Input: part model. Units: mm. Frame: model coordinates. Face numbers are marked on the shaded views. A direction names the side the tool comes from. Round coordinates to 2 decimals unless told otherwise and drop trailing zeros. Loops run counter-clockwise (first coordinate to the right, second up) from the corner with the lowest first, then second, coordinate; pieces in that order, holes last. Notation, with made-up numbers: (20, 72.5) - (64, 72.5) arc R16 ccw to (64, 81.5) - close; hole circle Ø7 at (80.25, -10.75). An arc over 180 degrees is marked (long way). Use CSV: the item, a comma, the result in double quotes. Start each with the question number.
1. Material intervals for probe 1 along X at (y, z) = (-58, 121.5); probe 2 along Y at (x, z) = (34.5, 263); probe 3 along Z at (x, y) = (143, -280.5), sorted ascending. Write a range as from..to.
2. Cut plane B-B (y = -93.5). Return loops of the section in (x, z) (3 decimals).
3. Pin query (flat end, axial travel): P1, Ø5, axis at x = 423.5, y = -401, coming from the +Z side; P2, Ø1, axis at y = -327.5, z = 31, coming from the -X side; P3, Ø5.5, axis at y = -265, z = 11, coming from the +X side. Return the tip coordinate at first contact, or that it passes through.
4. Pull-direction query (X, two-part tool) for the marked faces 1, 2 and 3; classes: +X half, -X half, draft (parallel to the pull), parting line (faces both ways), or undercut.
5. Cut plane C-C (x = 41). Return loops of the section in (y, z) (3 decimals).
6. Access query for the marked faces 4, 5 and 6. Directions: +Z, -Z, +X, -X, +Y, -Y. A direction counts if a zero-diameter tool reaches every point of the face in a straight line with its end or side. Return the directions, or none.
7. Cut plane A-A (z = 38.5). Return loops of the section in (x, y).
```python
from build123d import *

# Parameters (mm, degrees)
F0_W     = 520.7
F0_H     = 347.345
F1_DEPTH = 914.4
F2_T     = -11.90625
F4_DEPTH = 6.35
F5_W     = 496.8875
F5_H     = 3.175
F6_DEPTH = 366.396
F7_W     = 503.2375
F7_H     = 8.73125
F8_DEPTH = 914.4


with BuildPart() as f1:
    # F0 (on Front) → F1 (new body)
    with BuildSketch(Plane.XZ):
        with Locations((260.35, 173.6725)):
            Rectangle(F0_W, F0_H)
    extrude(amount=F1_DEPTH)

    # F2
    f2_openings = [f1.faces().sort_by_distance(p)[0] for p in [
        (260.35, -457.2, 347.345),
        (260.35, -457.2, 0),
    ]]
    offset(amount=F2_T, openings=f2_openings)

    # F3 (on face) → F4 (join)
    with BuildSketch(Plane.XZ.offset(914.4)):
        with BuildLine():
            ThreePointArc((-19.05, -6.35), (-15.330256, -15.330256), (-6.35, -19.05))
            Line((-6.35, -19.05), (527.05, -19.05))
            ThreePointArc((527.05, -19.05), (536.030256, -15.330256), (539.75, -6.35))
            Line((539.75, -6.35), (539.75, 353.695))
            ThreePointArc((539.75, 353.695), (536.030256, 362.675256), (527.05, 366.395))
            Line((527.05, 366.395), (-6.35, 366.395))
            ThreePointArc((-6.35, 366.395), (-15.330256, 362.675256), (-19.05, 353.695))
            Line((-19.05, 353.695), (-19.05, -6.35))
        make_face()
    extrude(amount=F4_DEPTH)

    # F5 (on face) → F6 (cut, through all)
    with BuildSketch(Plane.XY.offset(347.345)):
        with Locations((260.35, -10.31875)):
            Rectangle(F5_W, F5_H)
    extrude(amount=-F6_DEPTH, mode=Mode.SUBTRACT)

    # F7 (on face) → F8 (join, through all)
    with BuildSketch(Plane(origin=(0, 0, 0), x_dir=(-1, 0, 0), z_dir=(0, 1, 0))):
        with Locations((-260.35, 23.415625)):
            Rectangle(F7_W, F7_H)
    extrude(amount=-F8_DEPTH)


solid = f1.part
```
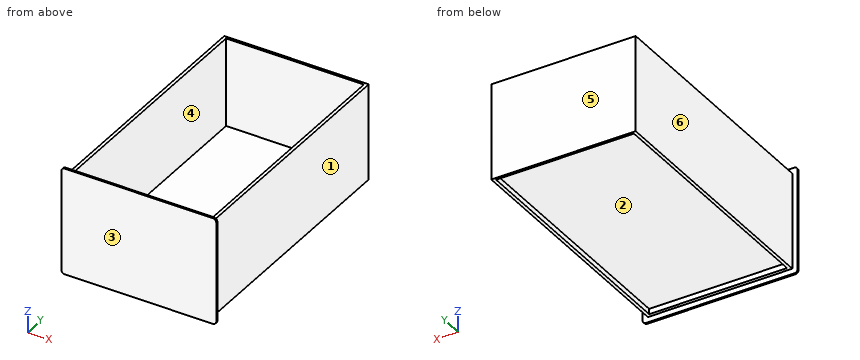
Established:
1,probe 1,"x = 0..11.91, 508.79..520.7"
1,probe 2,"y = -920.75..-902.49, -8.73..0"
1,probe 3,"z = 19.05..27.78"
2,outline,"(0, 0) - (11.906, 0) - (11.906, 19.05) - (508.794, 19.05) - (508.794, 0) - (520.7, 0) - (520.7, 347.345) - (508.794, 347.345) - (508.794, 27.781) - (11.906, 27.781) - (11.906, 347.345) - (0, 347.345) - close"
3,P1,"stops at z = 27.78"
3,P2,"stops at x = 0"
3,P3,"stops at x = 520.7"
4,face 1,"+X half"
4,face 2,"undercut"
4,face 3,"draft"
5,outline,"(-920.75, -19.05) - (-914.4, -19.05) - (-914.4, 0) - (-902.494, 0) - (-902.494, 19.05) - (-8.731, 19.05) - (-8.731, 0) - (0, 0) - (0, 347.345) - (-8.731, 347.345) - (-8.731, 27.781) - (-902.494, 27.781) - (-902.494, 347.345) - (-914.4, 347.345) - (-914.4, 366.395) - (-920.75, 366.395) - close"
6,face 4,"+Z"
6,face 5,"+Z, -Z, +X, -X, +Y"
6,face 6,"+Z, -Z, -X, +Y"
7,outline,"(-19.05, -920.75) - (539.75, -920.75) - (539.75, -914.4) - (520.7, -914.4) - (520.7, 0) - (0, 0) - (0, -914.4) - (-19.05, -914.4) - close; hole (11.91, -902.49) - (508.79, -902.49) - (508.79, -8.73) - (11.91, -8.73) - close"
